Geometry check sheet. Reference: drawing and pictorial views, mm from the part's lowest x, y, z. A direction names the side the tool comes from. Give positions to 0.01 mm unless a question says otherwise; leave off trailing zeros. Write each loop counter-clockwise with the first axis right and the second up, starting at its lowest first coordinate (ties: lowest second). Pieces come first, ordered by that corner, then holes. Notation, with made-up numbers: (27.5, -2) -> (58.5, -2) arc R24 ccw to (58.5, 15) -> close; hole circle Ø8 at (48.5, 40). An arc over 180 degrees is marked (long way). Use a Markdown table: item, result. Add a question column.
1. Release check for a two-part mould opening along Y. For the marked faces 1, 2, 3 and 4 record: released by +Y, released by -Y, zero draft, split by the parting line, or undercut.
2. Set-up check for the marked faces 5, 6 and 7: record each of +Z, -Z, +X, -X, +Y, -Y from which the full face is reachable in a straight line by a thin tool's end or side.
3. Scan lines: probe 1 along Y at (x, z) = (31.5, 36); probe 2 along X at (y, z) = (4.5, 63.5); probe 3 along X at (y, z) = (72.5, 25.5). Record each from-to range of solid material in increasing order. Write a range as [from, to].
4. Cross-section at D-D (x = 41.5). Enter the section's corners in (y, z).
5. Cross-section at C-C (z = 39.5). Enter the section's corners in (x, y) (1 decimal).
6. Cross-section at A-A (y = 48). Enter the section's corners in (x, z).
7. Cross-section at B-B (x = 101). Enter the section's corners in (y, z), then the cut area to 3 significant figures.
8. Gauge pin test, flat ends, axial feed: P1, Ø12.5, axis at x = 109, y = 14.5, coming from the -Z side; P2, Ø2, axis at x = 42, z = 47, coming from the +Y side; P3, Ø1, axis at y = 76.5, z = 19, coming from the +X side; P4, Ø7, axis at x = 7.5, z = 64.5, coming from the -Y side. Record the tip position at first contact, or that the pin passes through.
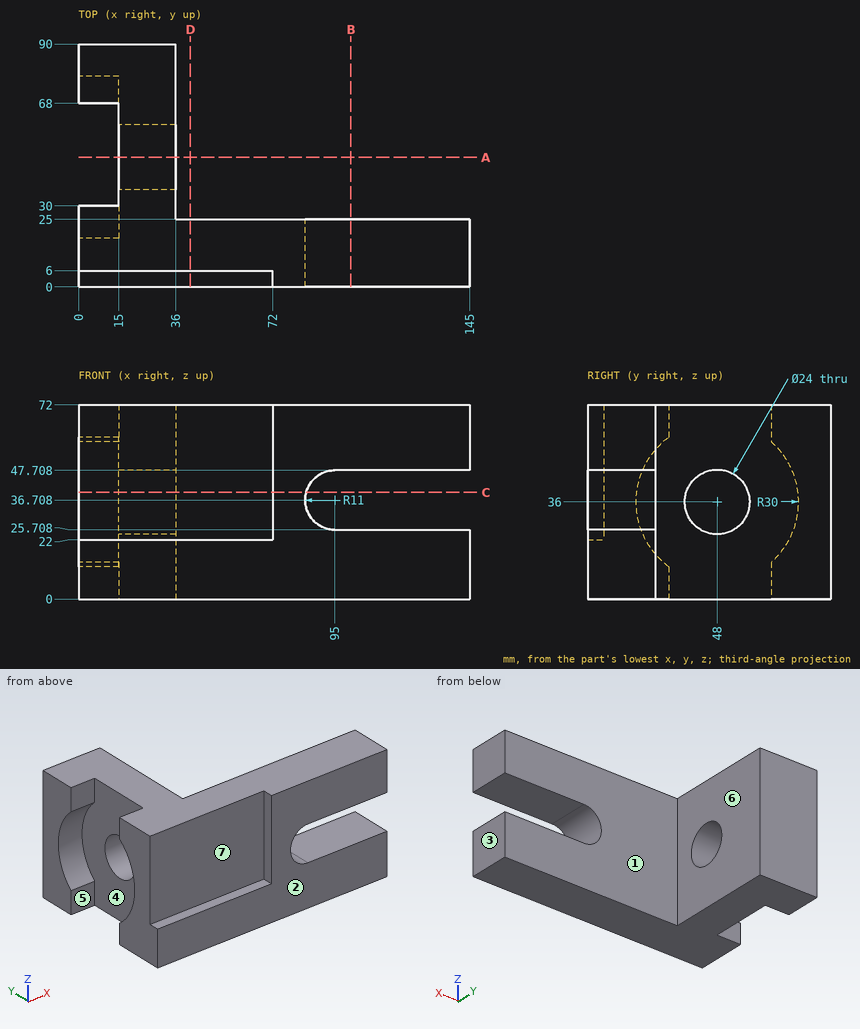
Worked answers:
| question | item | result |
|---|---|---|
| 1 | face 1 | released by +Y |
| 1 | face 2 | released by -Y |
| 1 | face 3 | zero draft |
| 1 | face 4 | undercut |
| 2 | face 5 | +Z, -Z, -X |
| 2 | face 6 | +Z, -Z, +X, +Y |
| 2 | face 7 | +Z, -X, -Y |
| 3 | probe 1 | y = [6, 36], [60, 90] |
| 3 | probe 2 | x = [72, 145] |
| 3 | probe 3 | x = [15, 36] |
| 4 | outline | (0, 0) -> (25, 0) -> (25, 72) -> (6, 72) -> (6, 22) -> (0, 22) -> close |
| 5 | outline | (0, 6) -> (72, 6) -> (72, 0) -> (84.4, 0) -> (84.4, 25) -> (36, 25) -> (36, 36.5) -> (15, 36.5) -> (15, 18.2) -> (0, 18.2) -> close; (0, 77.8) -> (15, 77.8) -> (15, 59.5) -> (36, 59.5) -> (36, 90) -> (0, 90) -> close |
| 6 | outline | (15, 0) -> (36, 0) -> (36, 24) -> (15, 24) -> close; (15, 48) -> (36, 48) -> (36, 72) -> (15, 72) -> close |
| 7 | outline | (0, 0) -> (25, 0) -> (25, 25.71) -> (0, 25.71) -> close; (0, 47.71) -> (25, 47.71) -> (25, 72) -> (0, 72) -> close |
| 7 | area | 1,250 mm² |
| 8 | P1 | stops at z = 0 |
| 8 | P2 | stops at y = 25 |
| 8 | P3 | stops at x = 36 |
| 8 | P4 | stops at y = 6 |
